Design review of the part built by this model. Coordinates are the model's own, in mm. Face numbers are marked on the shaded views. Coordinates: 2 decimals unless noted, no trailing zeros. Write item = value, one per line.
Autodesk Inventor part; units mm, degrees
ref_plane "YZ Plane" through (0, 0, 0) normal (1, 0, 0) x (0, 1, 0)
ref_plane "XZ Plane" through (0, 0, 0) normal (0, 1, 0) x (-1, 0, 0)
ref_plane "XY Plane" through (0, 0, 0) normal (0, 0, 1) x (1, 0, 0)
ref_plane "Work Plane1" through (0, 0, 0) normal (0, 0, -1) x (-1, 0, 0)
ref_plane "Work Plane3" through (-59.1654, 22.8024, -1.2767) normal (0, 0, 1) x (0, 1, 0)
sketch "Sketch4" plane through (-59.1654, 22.8024, -1.2767) normal (0, 0, 1) x (0, 1, 0)
  line L0 (0, 0.2578) -> (0, -48.4285) construction
  line L1 (-4.3051, -44.7422) -> (4.9106, -44.7422) construction
  circle A0 centre (0, -44.7422) radius 2.97
  circle A1 centre (0, 0) radius 25.1499 construction
  arc A2 (-4.4358, -46.9838) -> (4.4358, -46.9838) centre (0, -44.7422) ccw
  line L2 (0, -55.7616) -> (-22.5832, -11.0728)
  line L3 (0, -55.7616) -> (22.4465, -11.3432)
  arc A3 (22.4465, -11.3432) -> (-22.4465, -11.3432) centre (0, 0) ccw
  line L4 (0, 0) -> (0, -25.1499) construction
  line L5 (0, -41.7722) -> (0, -73.1545) construction
  point P0 (-22.8024, -59.1654)
  dimension "d9" = 5.94
  dimension "d8" = 45
  dimension "d10" = 2
extrude "Extrusion2" add sketch "Sketch4" along normal blind 2 contours L2 A3 L3 A2
fillet "Fillet2" radius 1.5 4 edges at (-9.4532, 22.8024, 0.7233) (-30.0019, 36.2436, 0.7233) (-84.3153, 22.8024, 0.7233) (-30.0019, 9.3612, 0.7233)
sketch "Sketch5" plane through (-59.1654, 22.8024, 0.7233) normal (0, 0, 1) x (1, 0, 0)
  line L0 (41.0298, 3.3493) -> (24.2777, 11.8149)
  line L1 (24.2777, -11.8149) -> (41.0298, -3.3493)
  line L2 (11.3432, -22.4465) -> (46.9838, -4.4358)
  line L3 (46.9838, 4.4358) -> (11.3432, 22.4465)
  arc A0 (46.9838, -4.4358) -> (46.9838, 4.4358) centre (44.7422, 0) ccw
  circle A1 centre (44.7422, 0) radius 2.97
  arc A2 (46.3073, -3.097) -> (46.3073, 3.097) centre (44.7422, 0) ccw
  line L4 (10.6667, 21.1078) -> (46.3073, 3.097)
  arc A3 (10.6667, 21.1078) -> (10.6667, -21.1078) centre (0, 0) ccw
  line L5 (46.3073, -3.097) -> (10.6667, -21.1078)
  line L6 (-0.2578, 0) -> (48.4285, 0) construction
  arc A4 (24.2777, -11.8149) -> (24.2777, 11.8149) centre (0, 0) ccw
  arc A5 (41.0298, 3.3493) -> (41.0298, -3.3493) centre (44.7422, 0) ccw
  line L7 (48.7042, -0.0038) -> (-50.8727, 0.004) construction
  point P0 (59.1654, -22.8024)
  point P1 (39.7422, -4)
  point P2 (39.7422, 4)
  point P3 (26.5473, 10.668)
  point P4 (26.5473, -10.668)
  dimension "d25" = 27
  dimension "d27" = 5
extrude "Extrusion3" cut sketch "Sketch5" against normal through all contours A5 L1 A4 L0
fillet "Fillet4" radius 1 4 edges at (-18.1356, 26.1517, -0.2767) (-18.1356, 19.4531, -0.2767) (-34.8877, 34.6173, -0.2767) (-34.8877, 10.9875, -0.2767)
fillet "Fillet5" radius 1 8 edges at (-33.56, 12.3687, 0.7233) (-32.1654, 22.8024, 0.7233) (-33.56, 33.2361, 0.7233) (-25.8107, 30.0303, 0.7233) (-18.6709, 26.073, 0.7233) (-19.4232, 22.8024, 0.7233) (-18.6709, 19.5318, 0.7233) (-25.8107, 15.5745, 0.7233)
sketch "Sketch6" plane through (-59.1654, 22.8024, -1.2767) normal (0, 0, -1) x (-1, 0, 0)
  line L0 (-47.2622, 0) -> (-42.2222, 0) construction
  circle A0 centre (-44.7422, 0) radius 4.17
  arc A1 (-46.9838, 4.4358) -> (-46.9838, -4.4358) centre (-44.7422, 0) ccw construction
  point P0 (-59.1654, -22.8024)
  dimension "d30" = 0.8
extrude "Extrusion4" add sketch "Sketch6" along normal blind 2.62
fillet "Fillet6" radius 1 1 edges at (-10.2532, 22.8024, -3.8967)
sketch "Sketch7" plane through (-14.4232, 22.8024, -1.2767) normal (0, 0, 1) x (1, 0, 0)
  circle A0 centre (0, 0) radius 2.97
  point P0 (14.4232, -22.8024)
extrude "Extrusion5" cut sketch "Sketch7" against normal blind 1.82
sketch "Sketch8" plane through (-14.4232, 22.8024, -3.8967) normal (0, 0, -1) x (-1, 0, 0)
  circle A0 centre (0, 0) radius 1.3
  point P0 (-14.4232, -22.8024)
hole "Hole1" at (-14.4232, 22.8024, -3.8967) direction (0, 0, 1) diameter 2.86 depth 1.82 countersink diameter 5.65 countersink angle 90
fillet "Fillet7" radius 0.5 1 edges at (-10.2532, 22.8024, -1.2767)
properties part number "trapdoor_servo" material "PET Plastic"
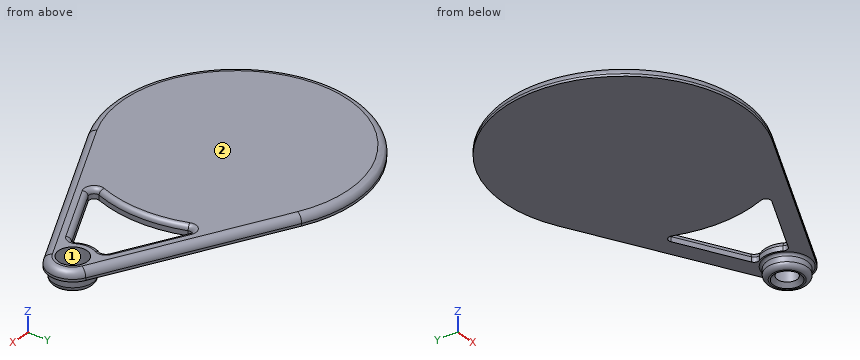
Q1. For P1, Ø5.5, axis at x = -14.42, y = 22.8, coming from the +Z side; P2, Ø1.5, axis at x = -73.5, z = -1.5, coming from the -Y side; P3, Ø2, axis at y = 5.5, z = -3, coming from the -X side; P4, Ø1, axis at x = -62.5, z = -0.5, coming from the -Y side, all flat-tipped, find the tip position at first contact; note any pin that passes through.
Check result:
P1 = -3.1
P2 = 1.66
P3 = through
P4 = -2.18
Q2. Wall thickness on line 1 (X direction, y = 25, z = -0.9) (3 decimals); line 2 (Z direction, x = -69, y = 36); line 3 (X direction, y = 28, z = -0.9): over which ranges is each line inside the solid? List them lowest first.
Check result:
line_1 = -84.219 to -32.255, -18.914 to -16.421, -12.425 to -9.965
line_2 = -1.28 to 0.72
line_3 = -83.77 to -32.67, -21.79 to -13.69
Q3. Consider section A-A, the plane y = 24. State how many separate pieces and enclosed holes the cut face has, and give its area (3 significant figures).
Check result:
separate_pieces = 3
enclosed_holes = 0
area = 119 mm²
Q4. The part is to be moulded in two halves that separate along X. For the marked faces 1 and 2, say which applies: +X half, -X half, draft (parallel to the pull), parting line (faces both ways), or undercut.
Check result:
face_1 = undercut
face_2 = draft
